```python
from build123d import *

# Parameters (mm, degrees)
F1_DEPTH = 2.54
F3_DEPTH = 5.08
F4_R     = 20.32
F5_DEPTH = 7.621
F6_R     = 2.54
F7_R     = 0.508


with BuildPart() as f1:
    # F0 (on Top) → F1 (new body)
    with BuildSketch(Plane.XY):
        Polygon((88.876464, 93.29783), (-12.723536, 93.29783), (-12.723536, -27.35217), (38.076464, -27.35217), (38.076464, -1.95217), (88.876464, -1.95217), align=None)
    extrude(amount=F1_DEPTH)

    # F2 (on face) → F3 (join)
    with BuildSketch(Plane(origin=(0, 0, 0), x_dir=(1, 0, 0), z_dir=(0, 0, -1))):
        Polygon((35.536464, -0.58783), (35.536464, 24.81217), (-10.183536, 24.81217), (-10.183536, -90.75783), (86.336464, -90.75783), (86.336464, -0.58783), align=None)
        Polygon((-7.643536, 22.27217), (32.996464, 22.27217), (32.996464, -3.12783), (83.796464, -3.12783), (83.796464, -88.21783), (-7.643536, -88.21783), align=None, mode=Mode.SUBTRACT)
    extrude(amount=F3_DEPTH)

    # F4 (on face) → F5 (cut, through all)
    with BuildSketch(Plane.XY.offset(2.54)):
        with Locations((38.076464, 66.62783)):
            Circle(F4_R)
    extrude(amount=-F5_DEPTH, mode=Mode.SUBTRACT)

    # F6
    f6_edges = [f1.edges().sort_by_distance(p)[0] for p in [
        (38.076464, -27.35217, 1.27),
        (35.536464, -24.81217, -2.54),
        (35.536464, 0.58783, -2.54),
        (38.076464, -1.95217, 1.27),
        (86.336464, 0.58783, -2.54),
        (88.876464, -1.95217, 1.27),
        (-12.723536, -27.35217, 1.27),
        (-10.183536, -24.81217, -2.54),
        (88.876464, 93.29783, 1.27),
        (86.336464, 90.75783, -2.54),
        (-12.723536, 93.29783, 1.27),
        (-10.183536, 90.75783, -2.54),
        (32.996464, 3.12783, -2.54),
        (32.996464, -22.27217, -2.54),
        (-7.643536, -22.27217, -2.54),
        (-7.643536, 88.21783, -2.54),
        (83.796464, 88.21783, -2.54),
        (83.796464, 3.12783, -2.54),
    ]]
    fillet(f6_edges, radius=F6_R)

    # F7
    f7_edges = [f1.edges().sort_by_distance(p)[0] for p in [
        (17.756464, 66.62783, 0),
        (17.756464, 66.62783, 2.54),
    ]]
    fillet(f7_edges, radius=F7_R)


solid = f1.part
```
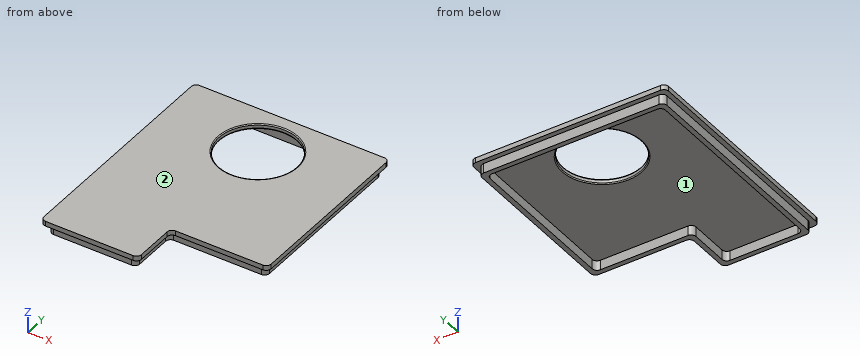
Design review of the part built by this model. Coordinates are the model's own, in mm. Face numbers are marked on the shaded views. Give positions to 0.01 mm unless a question says otherwise; leave off trailing zeros. Loops run counter-clockwise (first coordinate to the right, second up) from the corner with the lowest first, then second, coordinate; pieces in that order, holes last. Notation, with made-up numbers: M 22.5,-5 L 30.5,-5 A35 ccw 30.5,30 Z; hole C 47,5 d11. An arc over 180 degrees is marked long. Return JSON: item names as keys, results as strings. Group by question number.
Item 1: Mouldability with a two-part tool opening along Y and no side actions: class the marked faces 1 and 2 as released by +Y, released by -Y, zero draft, split by the parting line, or undercut.
Item 2: We need section A-A (z = -2.25). Give the boundary of the cut face in (x, y), and give its area (3 significant figures).
Item 3: Insertion check: pin 1 Ø1.5 at (y, z) = (-12.5, -2.5) entering from +X; pin 2 Ø1.5 at (x, z) = (37.5, -3) entering from +Y; pin 3 Ø1.5 at (y, z) = (-10, -2.5) entering from -X. Each pin has a flat end and moves straight along its axis. Give the tip position at first contact, or say it passes through.
Item 4: We need section C-C (x = 76.5). Give the boundary of the cut face in (y, z), and give its area (3 significant figures).
Item 5: We need section B-B (y = 24.5). Give the boundary of the cut face in (x, z).
Item 6: For probe 1 along X at (y, z) = (-16, -1.5); probe 2 along Y at (x, z) = (-5, -3); probe 3 along X at (y, z) = (83, -2.75), list the stretches that pass through material, from the lowest coordinate up.
Output:
{
 "1": {"face 1": "undercut", "face 2": "zero draft"},
 "2": {"outline": "M -10.18,-22.27 A2.54 ccw -7.64,-24.81 L 33,-24.81 A2.54 ccw 35.54,-22.27 L 35.54,-1.95 A2.54 cw 38.08,0.59 L 83.8,0.59 A2.54 ccw 86.34,3.13 L 86.34,88.22 A2.54 ccw 83.8,90.76 L -7.64,90.76 A2.54 ccw -10.18,88.22 Z; hole M -7.64,-19.73 A2.54 ccw -5.1,-22.27 L 30.46,-22.27 A2.54 ccw 33,-19.73 L 33,0.59 A2.54 cw 35.54,3.13 L 81.26,3.13 A2.54 ccw 83.8,5.67 L 83.8,85.68 A2.54 ccw 81.26,88.22 L -5.1,88.22 A2.54 ccw -7.64,85.68 Z", "area": "1,050 mm^2"},
 "3": {"pin 1": "stops at x = 35.54", "pin 2": "stops at y = 90.76", "pin 3": "stops at x = -10.18"},
 "4": {"outline": "M -1.95,0 L 0.59,0 L 0.59,-5.08 L 3.13,-5.08 L 3.13,0 L 88.22,0 L 88.22,-5.08 L 90.76,-5.08 L 90.76,0 L 93.3,0 L 93.3,2.54 L -1.95,2.54 Z", "area": "268 mm^2"},
 "5": {"outline": "M -12.72,0 L -10.18,0 L -10.18,-5.08 L -7.64,-5.08 L -7.64,0 L 83.8,0 L 83.8,-5.08 L 86.34,-5.08 L 86.34,0 L 88.88,0 L 88.88,2.54 L -12.72,2.54 Z"},
 "6": {"probe 1": "x = -10.18 to -7.64, 33 to 35.54", "probe 2": "y = -24.81 to -22.27, 88.22 to 90.76", "probe 3": "x = -10.18 to -7.64, 83.8 to 86.34"}
}
